Read the model definition and answer for the solid it produces. Units are mm, in the model's axes. A direction names the side the tool comes from. Coordinates: 2 decimals unless noted, no trailing zeros. Order: outer loops, then holes, each group sorted by start corner. A loop starts at its lowest first (then second) coordinate and runs counter-clockwise, first axis right, second up. Notation, with made-up numbers: (26.25, 10.25) -> (85.25, 10.25) arc R21 ccw to (85.25, 31.25) -> close; hole circle Ø3 at (50, 55). An arc over 180 degrees is marked (long way). Answer as a JSON object with one key per item and string values. Group by question number.
1) Section B-B on x = 13 is taken. Determine the outline of the cut face in (y, z).
2) Section A-A on y = -20.5 is taken. Count the separate pieces of the cut face and the enclosed holes in it, and give its area (3 significant figures).
3) Given pin 1 (2 mm diameter, centred on y = -13.5, z = -63.5, fed in from +X); pin 2 (5 mm diameter, centred on y = -21, z = -72.5, fed in from -X); pin 3 (4 mm diameter, centred on x = -5.78, z = -14.27, fed in from +Y); pin 4 (8 mm diameter, centred on x = 42, y = -20.5, fed in from -Z), each flat-ended and moving along its own axis, determine where each tip first touches the part or whether it passes through.
4) Section D-D on x = 26 is taken. Determine the outline of the cut face in (y, z), and give its area (3 significant figures).
5) Section C-C on z = -36 is taken. Determine the outline of the cut face in (x, y).
6) A tool of negligible diameter and unlimited length cuts with its end or side. For faces 1 (the flat face through (13.408, -12.522, -75.559)), 2 (the cylindrical face through (41.52, -12.52, -115.52)), from which of +Z, -Z, +X, -X, +Y, -Y can it reach the whole face along a straight path? Write none if from no direction.
7) Consider L1, parallel to X at y = -5, z = -114.3 (1 decimal); L2, parallel to Z at x = 1.5, y = -23.5; L3, parallel to Z at x = 44.5, y = -1. Determine where each line is inside the solid, lowest interval first.
from build123d import *

# Parameters (mm, degrees)
F0_R     = 2.6007380418
F1_DEPTH = 25.4


with BuildPart() as f1:
    # F0 (on Front) → F1 (new body)
    with BuildSketch(Plane.XZ):
        with BuildLine():
            Line((-15.8738293827, -50.6072158518), (-15.4295331686, -47.0656819632))
            ThreePointArc((-15.4295331686, -47.0656819632), (-15.751531428, -48.8239224018), (-15.8738293827, -50.6072158518))
        make_face()
        with BuildLine():
            Line((-15.5233638186, -54.1227700425), (-15.8738293827, -50.6072158518))
            ThreePointArc((-15.8738293827, -50.6072158518), (-15.7966995144, -52.3747728257), (-15.5233638186, -54.1227700425))
        make_face()
        with BuildLine():
            ThreePointArc((15.5879837413, -53.8050603789), (15.7958662647, -52.38310895), (15.874308373, -50.9481846156))
            Line((15.874308373, -50.9481846156), (15.5879837413, -53.8050603789))
        make_face()
        with BuildLine():
            ThreePointArc((15.875, -50.8), (15.7438070308, -48.7632955104), (15.352396513, -46.7602541779))
            Line((15.352396513, -46.7602541779), (15.874308373, -50.9481846156))
            ThreePointArc((15.874308373, -50.9481846156), (15.8748270923, -50.8740931148), (15.875, -50.8))
        make_face()
        with BuildLine():
            Line((0.6778573649, -123.8008491406), (0, -123.825))
            ThreePointArc((0, -123.825), (0.3391437273, -123.8189603703), (0.6778573649, -123.8008491406))
        make_face()
        with BuildLine():
            ThreePointArc((9.525, 0), (6.7351920908, -6.7351920908), (0, -9.525))
            Line((0, -9.525), (0, -34.925))
            ThreePointArc((0, -34.925), (9.6923851573, -38.227279731), (15.352396513, -46.7602541779))
            Line((15.352396513, -46.7602541779), (9.525, 0))
        make_face()
        with BuildLine():
            Line((0, -104.775), (0, -66.675))
            ThreePointArc((0, -66.675), (-9.9816494272, -63.14432257), (-15.5233638186, -54.1227700425))
            Line((-15.5233638186, -54.1227700425), (-9.5249974039, -114.2929674737))
            ThreePointArc((-9.5249974039, -114.2929674737), (-6.7327052582, -107.5623219944), (0, -104.775))
        make_face()
        with BuildLine():
            Line((36.5125, -114.3), (9.525, -114.3))
            ThreePointArc((9.525, -114.3), (6.9707322571, -120.7911105983), (0.6778573649, -123.8008491406))
            Line((0.6778573649, -123.8008491406), (44.5940537667, -122.236192712))
            ThreePointArc((44.5940537667, -122.236192712), (38.888503822, -119.9633617677), (36.5125, -114.3))
        make_face()
        with BuildLine():
            ThreePointArc((52.3875, -114.3), (50.0626600757, -108.6873399243), (44.45, -106.3625))
            ThreePointArc((44.45, -106.3625), (38.8373399243, -108.6873399243), (36.5125, -114.3))
            ThreePointArc((36.5125, -114.3), (38.888503822, -119.9633617677), (44.5940537667, -122.236192712))
            ThreePointArc((44.5940537667, -122.236192712), (50.1133617677, -119.861496178), (52.3875, -114.3))
        make_face()
        with BuildLine():
            ThreePointArc((47.625, -114.3), (44.45, -117.475), (41.275, -114.3))
            ThreePointArc((41.275, -114.3), (44.45, -111.125), (47.625, -114.3))
        make_face(mode=Mode.SUBTRACT)
        with BuildLine():
            ThreePointArc((-9.525, 0), (-6.7351920908, -6.7351920908), (0, -9.525))
            ThreePointArc((0, -9.525), (6.7351920908, -6.7351920908), (9.525, 0))
            ThreePointArc((9.525, 0), (0, 9.525), (-9.525, 0))
        make_face()
        with BuildLine():
            ThreePointArc((3.175, 0), (2.2450640303, -2.2450640303), (0, -3.175))
            ThreePointArc((0, -3.175), (-2.2450640303, 2.2450640303), (3.175, 0))
        make_face(mode=Mode.SUBTRACT)
        with BuildLine():
            Line((0, -111.125), (0, -104.775))
            ThreePointArc((0, -104.775), (-6.7327052582, -107.5623219944), (-9.5249974039, -114.2929674737))
            ThreePointArc((-9.5249974039, -114.2929674737), (-6.7376780056, -121.0327052582), (0, -123.825))
            Line((0, -123.825), (0.6778573649, -123.8008491406))
            ThreePointArc((0.6778573649, -123.8008491406), (6.9707322571, -120.7911105983), (9.525, -114.3))
            Line((9.525, -114.3), (3.175, -114.3))
            ThreePointArc((3.175, -114.3), (-2.2450640303, -116.5450640303), (0, -111.125))
        make_face()
        with BuildLine():
            ThreePointArc((15.5879837413, -53.8050603789), (10.1071828787, -63.0417514783), (0, -66.675))
            Line((0, -66.675), (0, -104.775))
            ThreePointArc((0, -104.775), (0.3399618281, -104.7810688123), (0.6794904459, -104.7992675159))
            ThreePointArc((0.6794904459, -104.7992675159), (6.9712901065, -107.8094885216), (9.525, -114.3))
            Line((9.525, -114.3), (36.5125, -114.3))
            ThreePointArc((36.5125, -114.3), (38.8373399243, -108.6873399243), (44.45, -106.3625))
            Line((44.45, -106.3625), (18.914480682, -105.4505171672))
            ThreePointArc((18.914480682, -105.4505171672), (13.2086857771, -102.7332860354), (11.2876656625, -96.7125616404))
            Line((11.2876656625, -96.7125616404), (15.5879837413, -53.8050603789))
        make_face()
        with BuildLine():
            Line((0, -34.925), (0, -9.525))
            ThreePointArc((0, -9.525), (-6.7351920908, -6.7351920908), (-9.525, 0))
            Line((-9.525, 0), (-15.4295331686, -47.0656819632))
            ThreePointArc((-15.4295331686, -47.0656819632), (-9.8166523359, -38.3240646877), (0, -34.925))
        make_face()
        with Locations((-5.7757380418, -14.2748)):
            Circle(F0_R, mode=Mode.SUBTRACT)
        with BuildLine():
            Line((0, -47.625), (0, -34.925))
            ThreePointArc((0, -34.925), (-9.8166523359, -38.3240646877), (-15.4295331686, -47.0656819632))
            Line((-15.4295331686, -47.0656819632), (-15.8738293827, -50.6072158518))
            Line((-15.8738293827, -50.6072158518), (-15.5233638186, -54.1227700425))
            ThreePointArc((-15.5233638186, -54.1227700425), (-9.9816494272, -63.14432257), (0, -66.675))
            Line((0, -66.675), (0, -53.975))
            ThreePointArc((0, -53.975), (-3.175, -50.8), (0, -47.625))
        make_face()
        with BuildLine():
            ThreePointArc((15.352396513, -46.7602541779), (9.6923851573, -38.227279731), (0, -34.925))
            Line((0, -34.925), (0, -47.625))
            ThreePointArc((0, -47.625), (2.2450640303, -48.5549359697), (3.175, -50.8))
            ThreePointArc((3.175, -50.8), (2.2450640303, -53.0450640303), (0, -53.975))
            Line((0, -53.975), (0, -66.675))
            ThreePointArc((0, -66.675), (10.1071828787, -63.0417514783), (15.5879837413, -53.8050603789))
            Line((15.5879837413, -53.8050603789), (15.874308373, -50.9481846156))
            Line((15.874308373, -50.9481846156), (15.352396513, -46.7602541779))
        make_face()
        with BuildLine():
            Line((0.6794904459, -104.7992675159), (0, -104.775))
            Line((0, -104.775), (0, -111.125))
            ThreePointArc((0, -111.125), (2.2450640303, -112.0549359697), (3.175, -114.3))
            Line((3.175, -114.3), (9.525, -114.3))
            ThreePointArc((9.525, -114.3), (6.9712901065, -107.8094885216), (0.6794904459, -104.7992675159))
        make_face()
    extrude(amount=F1_DEPTH)


solid = f1.part
Worked answers:
{
 "1": {"outline": "(-25.4, -123.36) -> (0, -123.36) -> (0, -102.48) -> (-25.4, -102.48) -> close; (-25.4, -79.63) -> (0, -79.63) -> (0, -27.88) -> (-25.4, -27.88) -> close"},
 "2": {"separate pieces": "1", "enclosed holes": "6", "area": "3,770 mm²"},
 "3": {"pin 1": "stops at x = 14.72", "pin 2": "stops at x = -13.94", "pin 3": "passes through", "pin 4": "stops at z = -122.47"},
 "4": {"outline": "(-25.4, -122.9) -> (0, -122.9) -> (0, -105.7) -> (-25.4, -105.7) -> close", "area": "437 mm²"},
 "5": {"outline": "(-14.04, -25.4) -> (14.01, -25.4) -> (14.01, 0) -> (-14.04, 0) -> close"},
 "6": {"face 1": "+X, +Y, -Y", "face 2": "+Y, -Y"},
 "7": {"L1": "x = -9.5 to -3.2, 3.2 to 41.3, 47.6 to 52.4", "L2": "z = -123.77 to -117.1, -111.5 to -53.6, -48 to -2.8, 2.8 to 9.41", "L3": "z = -122.24 to -117.47, -111.13 to -106.36"}
}
